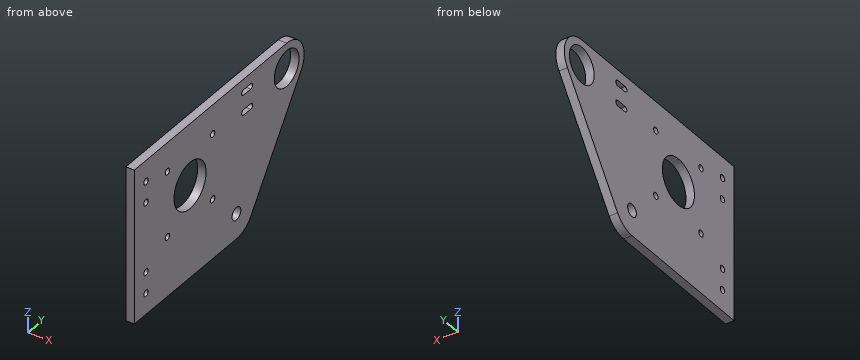
from build123d import *

# Parameters (mm, degrees)
SKETCH_1_R      = 3
SKETCH_1_R_2    = 8.5
SKETCH_1_R_3    = 11
SKETCH_1_R_4    = 1.5
EXTRUDE_1_DEPTH = 4


with BuildPart() as part:
    # 草图1 → 凸台-拉伸1 (new body)
    with BuildSketch(Plane(origin=(0, 0, 0), x_dir=(0, 0, -1), z_dir=(1, 0, 0))):
        with BuildLine():
            Line((-42.273933648, 44.23702673), (6.8812, 9.83102673))
            ThreePointArc((6.8812, 9.83102673), (10.643645992, 5.541913027), (12, 0))
            Line((12, 0), (12, -70))
            Line((12, -70), (-61.155133648, -70))
            Line((-61.155133648, -70), (-61.155133648, 34.406))
            ThreePointArc((-61.155133648, 34.406), (-54.697046676, 45.049645992), (-42.273933648, 44.23702673))
        make_face()
        Circle(SKETCH_1_R, mode=Mode.SUBTRACT)
        with Locations((-49.155133648, 34.406)):
            Circle(SKETCH_1_R_2, mode=Mode.SUBTRACT)
        with Locations((-31.819805153, -31.819805153)):
            Circle(SKETCH_1_R_3, mode=Mode.SUBTRACT)
        with Locations((2, -62)):
            Circle(SKETCH_1_R_4, mode=Mode.SUBTRACT)
        with Locations((-8, -62)):
            Circle(SKETCH_1_R_4, mode=Mode.SUBTRACT)
        with Locations((-41.155133648, -62)):
            Circle(SKETCH_1_R_4, mode=Mode.SUBTRACT)
        with Locations((-51.155133648, -62)):
            Circle(SKETCH_1_R_4, mode=Mode.SUBTRACT)
        with Locations((-16.319805153, -16.319805153)):
            Circle(SKETCH_1_R_4, mode=Mode.SUBTRACT)
        with Locations((-16.319805153, -47.319805147)):
            Circle(SKETCH_1_R_4, mode=Mode.SUBTRACT)
        with Locations((-47.319805147, -47.319805147)):
            Circle(SKETCH_1_R_4, mode=Mode.SUBTRACT)
        with Locations((-47.319805147, -16.319805153)):
            Circle(SKETCH_1_R_4, mode=Mode.SUBTRACT)
        with BuildLine():
            Line((-53.555133648, 9.83102673), (-53.555133648, 4.83102673))
            ThreePointArc((-53.555133648, 4.83102673), (-54.855133648, 3.53102673), (-56.155133648, 4.83102673))
            Line((-56.155133648, 4.83102673), (-56.155133648, 9.83102673))
            ThreePointArc((-56.155133648, 9.83102673), (-54.855133648, 11.13102673), (-53.555133648, 9.83102673))
        make_face(mode=Mode.SUBTRACT)
        with BuildLine():
            Line((-44.055133648, 9.83102673), (-44.055133648, 4.83102673))
            ThreePointArc((-44.055133648, 4.83102673), (-45.355133648, 3.53102673), (-46.655133648, 4.83102673))
            Line((-46.655133648, 4.83102673), (-46.655133648, 9.83102673))
            ThreePointArc((-46.655133648, 9.83102673), (-45.355133648, 11.13102673), (-44.055133648, 9.83102673))
        make_face(mode=Mode.SUBTRACT)
    extrude(amount=EXTRUDE_1_DEPTH)


solid = part.part
Verification items for the finished model (mm, model axes). Coordinates: 2 decimals unless noted, no trailing zeros. Order: outer loops, then holes, each group sorted by start corner. A loop starts at its lowest first (then second) coordinate and runs counter-clockwise, first axis right, second up.
Item 1: Section check B-B, the plane z = 8. Enter the section's corners in (x, y).
Filled in:
outline: (0, -70) - (4, -70) - (4, -63.5) - (0, -63.5) - close; (0, -60.5) - (4, -60.5) - (4, 20.25) - (0, 20.25) - close
Item 2: Section check C-C, the plane y = 8.5. Enter the section's corners in (x, z), then the cut area to 3 significant figures.
Filled in:
outline: (0, -8.47) - (4, -8.47) - (4, 44.06) - (0, 44.06) - close; (0, 46.66) - (4, 46.66) - (4, 53.56) - (0, 53.56) - close; (0, 56.16) - (4, 56.16) - (4, 61.16) - (0, 61.16) - close
area: 258 mm2
Item 3: Section check A-A, the plane y = -62. Enter the section's corners in (x, z).
Filled in:
outline: (0, -12) - (4, -12) - (4, -3.5) - (0, -3.5) - close; (0, -0.5) - (4, -0.5) - (4, 6.5) - (0, 6.5) - close; (0, 9.5) - (4, 9.5) - (4, 39.66) - (0, 39.66) - close; (0, 42.66) - (4, 42.66) - (4, 49.66) - (0, 49.66) - close; (0, 52.66) - (4, 52.66) - (4, 61.16) - (0, 61.16) - close
Item 4: Section check D-D, the plane x = 2.5. Give the number of separate pieces and of enclosed holes in the cut face, then the cut area to 3 significant figures.
Filled in:
separate pieces: 1
enclosed holes: 13
area: 6,600 mm2
Item 5: Depth check by flat-ended pin: pin 1 (1.5 mm diameter, centred on x = 1.5, z = 27, fed in from +Y); pin 2 (1 mm diameter, centred on x = 2, z = 19, fed in from +Y); pin 3 (2 mm diameter, centred on x = 3, z = 7.5, fed in from +Y). Enter the tip coordinate at first touch or a pass-through.
Filled in:
pin 1: stops at y = 34.07
pin 2: stops at y = 28.3
pin 3: stops at y = 20.6
Item 6: Material ranges on L1, parallel to Y at x = 1.35, z = -2; L2, parallel to Z at x = 2.25, y = -63; L3, parallel to Y at x = 3, z = 52.5, recorded low to high.
Filled in:
L1: y = -70 to -63.5, -60.5 to -2.24, 2.24 to 13.25
L2: z = -12 to -3.12, -0.88 to 6.88, 9.12 to 40.04, 42.27 to 50.04, 52.27 to 61.16
L3: y = -70 to -62.66, -61.34 to 26.59, 42.22 to 45.93
